Geometry check sheet. Reference: the model listing, model coordinates, mm. Face numbers are marked on the shaded views. A direction names the side the tool comes from. Round coordinates to 2 decimals unless told otherwise and drop trailing zeros. Write each loop counter-clockwise with the first axis right and the second up, starting at its lowest first coordinate (ties: lowest second). Pieces come first, ordered by that corner, then holes. Notation, with made-up numbers: M 31,11 L 82,11 A25 cw 82,32 Z; hole C 29.5,-15.5 d5. An arc over 180 degrees is marked long. Answer in a Markdown table with one row per item. Add a question column.
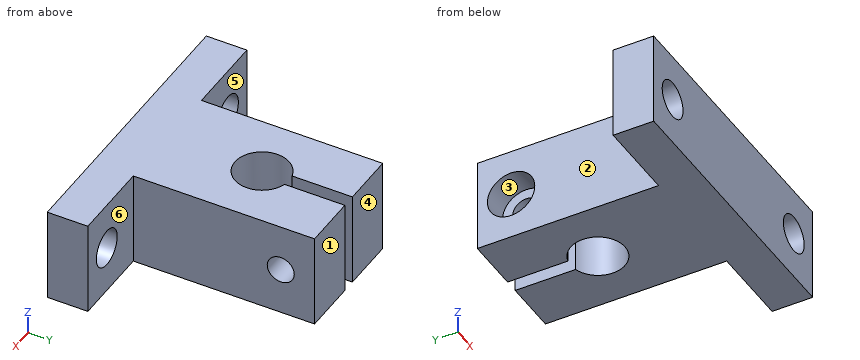
from build123d import *

# Parameters (mm, degrees)
EXTRUDE_1_DEPTH     = 14
SKETCH_2_R          = 4
SKETCH_2_W          = 2
SKETCH_2_H          = 8.927016654
CUT_EXTRUDE_2_DEPTH = 14
CUT_EXTRUDE_3_REACH = 34.8
SKETCH_4_R          = 2.75
SKETCH_5_R          = 2
CUT_EXTRUDE_4_DEPTH = 18
SKETCH_6_R          = 3.5
CUT_EXTRUDE_5_DEPTH = 4


with BuildPart() as part:
    # 草图1 → 凸台-拉伸1 (new body)
    with BuildSketch(Plane.XY):
        Polygon((21, 0), (-21, 0), (-21, 6), (-9, 6), (-9, 32.8), (9, 32.8), (9, 6), (21, 6), align=None)
    extrude(amount=EXTRUDE_1_DEPTH)

    # 草图2 → 切除-拉伸2 (cut)
    with BuildSketch(Plane(origin=(0, 0, 0), x_dir=(-1, 0, 0), z_dir=(0, 0, -1))):
        with Locations((0, 20)):
            Circle(SKETCH_2_R)
        with Locations((0, 28.336491673)):
            Rectangle(SKETCH_2_W, SKETCH_2_H)
    extrude(amount=-CUT_EXTRUDE_2_DEPTH, mode=Mode.SUBTRACT)

    # 草图4 → 切除-拉伸3 (cut, up to next)
    with BuildSketch(Plane.XZ, mode=Mode.PRIVATE) as cut_extrude_3_sk1:
        with Locations((16, 7)):
            Circle(SKETCH_4_R)
    cut_extrude_3_tool1 = extrude(cut_extrude_3_sk1.sketch, amount=-CUT_EXTRUDE_3_REACH, mode=Mode.PRIVATE) & part.part
    add(cut_extrude_3_tool1.solids().sort_by_distance((16, 0, 7))[0], mode=Mode.SUBTRACT)
    # 草图4 → 切除-拉伸3 (cut, up to next)
    with BuildSketch(Plane.XZ, mode=Mode.PRIVATE) as cut_extrude_3_sk2:
        with Locations((-16, 7)):
            Circle(SKETCH_4_R)
    cut_extrude_3_tool2 = extrude(cut_extrude_3_sk2.sketch, amount=-CUT_EXTRUDE_3_REACH, mode=Mode.PRIVATE) & part.part
    add(cut_extrude_3_tool2.solids().sort_by_distance((-16, 0, 7))[0], mode=Mode.SUBTRACT)

    # 草图5 → 切除-拉伸4 (cut)
    with BuildSketch(Plane.ZY.offset(9)):
        with Locations((7, 27.8)):
            Circle(SKETCH_5_R)
    extrude(amount=-CUT_EXTRUDE_4_DEPTH, mode=Mode.SUBTRACT)

    # 草图6 → 切除-拉伸5 (cut)
    with BuildSketch(Plane.ZY.offset(9)):
        with Locations((7, 27.8)):
            Circle(SKETCH_6_R)
    extrude(amount=-CUT_EXTRUDE_5_DEPTH, mode=Mode.SUBTRACT)


solid = part.part
Item 1: Section check A-A, the plane x = -16. Record the boundary of the cut face in (y, z), and give its area (3 significant figures).
Item 2: Access from +Z, -Z, +X, -X, +Y, -Y to the whole of each face (thin tool, end or side, straight path). Record for the marked faces 4, 5 and 6.
Item 3: Section check C-C, the plane y = 5. Record the boundary of the cut face in (x, z), and give its area (3 significant figures).
Item 4: Scan lines: probe 1 along X at (y, z) = (20, 6.25); probe 2 along Y at (x, z) = (-6.9, 7); probe 3 along Y at (x, z) = (-2.5, 7.5). Record each from-to range of solid material in increasing order. Write a range as from..to.
Item 5: Mould release check, pull along Y, two halves, no side actions. Record for the marked faces 1, 2 and 3: +Y half, -Y half, draft (parallel to the pull), parting line (faces both ways), or undercut.
Item 6: Gauge pin test, flat ends, axial feed: pin 1 Ø5.5 at (y, z) = (27.8, 7) entering from -X; pin 2 Ø8 at (x, z) = (-15.5, 2) entering from +Y; pin 3 Ø4.5 at (y, z) = (27.8, 7) entering from +X. Record the tip position at first contact, or that the pin passes through.
Item 7: Section check B-B, the plane z = 6. Give the number of separate pieces and of enclosed holes in the cut face, and give its area (3 significant figures).
Item 8: Section check D-D, the plane x = 3. Record the boundary of the cut face in (y, z).
Result sheet:
| question | item | result |
|---|---|---|
| 1 | outline | M 0,0 L 6,0 L 6,4.25 L 0,4.25 Z; M 0,9.75 L 6,9.75 L 6,14 L 0,14 Z |
| 1 | area | 51.0 mm^2 |
| 2 | face 4 | +Z, -Z, +X, -X, +Y |
| 2 | face 5 | +Z, -Z, -X, +Y |
| 2 | face 6 | +Z, -Z, +X, +Y |
| 3 | outline | M -21,0 L 21,0 L 21,14 L -21,14 Z; hole C -16,7 d5.5; hole C 16,7 d5.5 |
| 3 | area | 540 mm^2 |
| 4 | probe 1 | x = -9..-4, 4..9 |
| 4 | probe 2 | y = 0..24.3, 31.3..32.8 |
| 4 | probe 3 | y = 0..16.88, 23.12..25.86, 29.74..32.8 |
| 5 | face 1 | +Y half |
| 5 | face 2 | draft |
| 5 | face 3 | undercut |
| 6 | pin 1 | stops at x = -5 |
| 6 | pin 2 | stops at y = 6 |
| 6 | pin 3 | stops at x = 9 |
| 7 | separate pieces | 5 |
| 7 | enclosed holes | 0 |
| 7 | area | 537 mm^2 |
| 8 | outline | M 0,0 L 17.35,0 L 17.35,14 L 0,14 Z; M 22.65,0 L 32.8,0 L 32.8,14 L 22.65,14 Z; hole C 27.8,7 d4 |
